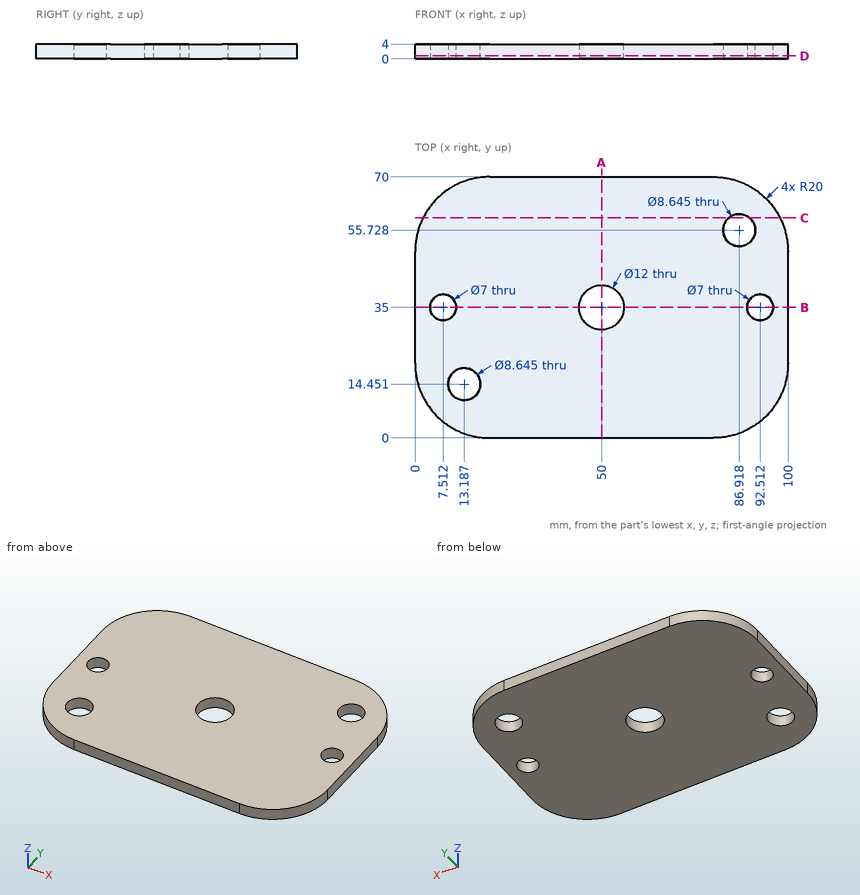
The drawing under review shows one solid part. Ordinate dimensions are in mm from its lowest x, y, z. Give positions to 0.01 mm unless a question says otherwise; leave off trailing zeros. Write each loop counter-clockwise with the first axis right and the second up, starting at its lowest first coordinate (ties: lowest second). Pieces come first, ordered by that corner, then holes. Notation, with made-up numbers: (-39, 53.25) - (10, 53.25) arc R14 ccw to (10, 65.25) - close; hole circle Ø1 at (79.25, 7.5). An arc over 180 degrees is marked (long way). Answer in a Markdown table with one row per item. Add a question column.
1. Insertion check: P1, Ø1.5, axis at y = 11, z = 2.5, coming from the -X side. The pin has a flat end and moves straight along its axis. Give the tip position at first contact, or say it passes through.
2. We need section A-A on x = 50. Write out the cut boundary in (y, z).
3. Wall thickness on line 1 along X through (y, z) = (35, 2.6); line 2 along X through (y, z) = (38, 3.5) (1 decimal); line 3 along X through (y, z) = (50.5, 1.7): over which ranges is each line inside the solid? List them lowest first. Write a range as [from, to].
4. We need section D-D on z = 0.8. Write out the cut boundary in (x, y) (1 decimal), then the cut area to 3 significant figures.
5. We need section B-B on y = 35. Write out the cut boundary in (x, z), then the cut area to 3 significant figures.
6. We need section C-C on y = 59. Write out the cut boundary in (x, z), then the cut area to 3 significant figures.
Ans:
| question | item | result |
|---|---|---|
| 1 | P1 | stops at x = 1.78 |
| 2 | outline | (0, 0) - (29, 0) - (29, 4) - (0, 4) - close; (41, 0) - (70, 0) - (70, 4) - (41, 4) - close |
| 3 | line 1 | x = [0, 4.01], [11.01, 44], [56, 89.01], [96.01, 100] |
| 3 | line 2 | x = [0, 5.7], [9.3, 44.8], [55.2, 90.7], [94.3, 100] |
| 3 | line 3 | x = [0.01, 99.99] |
| 4 | outline | (0, 20) arc R20 ccw to (20, 0) - (80, 0) arc R20 ccw to (100, 20) - (100, 50) arc R20 ccw to (80, 70) - (20, 70) arc R20 ccw to (0, 50) - close; hole circle Ø7 at (7.5, 35); hole circle Ø8.6 at (13.2, 14.5); hole circle Ø12 at (50, 35); hole circle Ø8.6 at (86.9, 55.7); hole circle Ø7 at (92.5, 35) |
| 4 | area | 6,350 mm^2 |
| 5 | outline | (0, 0) - (4.01, 0) - (4.01, 4) - (0, 4) - close; (11.01, 0) - (44, 0) - (44, 4) - (11.01, 4) - close; (56, 0) - (89.01, 0) - (89.01, 4) - (56, 4) - close; (96.01, 0) - (100, 0) - (100, 4) - (96.01, 4) - close |
| 5 | area | 296 mm^2 |
| 6 | outline | (2.14, 0) - (84.09, 0) - (84.09, 4) - (2.14, 4) - close; (89.74, 0) - (97.86, 0) - (97.86, 4) - (89.74, 4) - close |
| 6 | area | 360 mm^2 |
